Source: CAD feature listing. Evaluate the final solid. Frame: model axes, mm. A direction names the side the tool comes from. Round coordinates to 2 decimals unless told otherwise and drop trailing zeros. Write each loop counter-clockwise with the first axis right and the second up, starting at its lowest first coordinate (ties: lowest second). Pieces come first, ordered by that corner, then holes. Notation, with made-up numbers: (-10.75, -31.5) -> (3.25, -31.5) arc R20 ccw to (3.25, -6.5) -> close; hole circle Ø9 at (89, 87). An arc over 180 degrees is marked (long way). Return JSON: item names as keys, results as strings. Group by question number.
from build123d import *

# Parameters (mm, degrees)
F0_W     = 5.08
F0_H     = 5.08
F1_DEPTH = 5.08


# Not quite as in the source:
# - a feature names something its author has since deleted; it is built from what else it names


with BuildPart() as f1:
    # F0 (on Front) → F1 (new body)
    with BuildSketch(Plane.XZ):
        Polygon((0, 5.08), (0, 10.16), (-76.2, 10.16), (-76.2, 5.08), (-71.12, 5.08), (-71.12, 0), (-66.04, 0), (-66.04, -5.08), (-60.96, -5.08), (-60.96, -10.16), (-55.88, -10.16), (-55.88, -15.24), (-20.32, -15.24), (-20.32, -10.16), (-15.24, -10.16), (-15.24, -5.08), (-10.16, -5.08), (-10.16, 0), (-5.08, 0), (-5.08, 5.08), align=None)
        with Locations((-48.26, -7.62)):
            Rectangle(F0_W, F0_H, mode=Mode.SUBTRACT)
        with Locations((-38.1, -7.62)):
            Rectangle(F0_W, F0_H, mode=Mode.SUBTRACT)
        with Locations((-58.42, 2.54)):
            Rectangle(F0_W, F0_H, mode=Mode.SUBTRACT)
        with Locations((-48.26, 2.54)):
            Rectangle(F0_W, F0_H, mode=Mode.SUBTRACT)
        Polygon((76.2, 10.16), (0, 10.16), (0, 5.08), (5.08, 5.08), (5.08, 0), (10.16, 0), (10.16, -5.08), (15.24, -5.08), (15.24, -10.16), (20.32, -10.16), (55.88, -10.16), (60.96, -10.16), (60.96, -5.08), (66.04, -5.08), (66.04, 0), (71.12, 0), (71.12, 5.08), (76.2, 5.08), align=None)
        with Locations((17.78, 2.54)):
            Rectangle(F0_W, F0_H, mode=Mode.SUBTRACT)
        with Locations((27.94, 2.54)):
            Rectangle(F0_W, F0_H, mode=Mode.SUBTRACT)
    extrude(amount=-F1_DEPTH)


solid = f1.part
Item 1: Cut plane D-D on x = -38.5. Output: boundary loops of the cut face in (y, z).
Item 2: Material intervals for probe 1 along X at (y, z) = (2.55, -5.5); probe 2 along X at (y, z) = (4.45, -0.5); probe 3 along X at (y, z) = (1.05, -12.25), sorted ascending.
Item 3: Pull-direction query (X, two-part tool) for faces 6 (the flat face through (76.2, 3, 8)), 7 (the flat face through (-38, 3, -5.08)), 8 (the flat face through (74, 3, 5.08)); classes: +X half, -X half, draft (parallel to the pull), parting line (faces both ways), or undercut.
Item 4: Cut plane B-B on z = 2.25. Output: boundary loops of the cut face in (x, y), and give its area (3 significant figures).
Item 5: First-contact query: pin 1 Ø2 at (y, z) = (2, -3) entering from +X; pin 2 Ø1.5 at (x, y) = (-8.5, 2.5) entering from -Z; pin 3 Ø3 at (y, z) = (2.5, 1) entering from -X. Flat tips, straight axial feed; report the tip coordinate or a pass-through.
Item 6: Cut plane C-C on y = 3.2. Give the number of separate pieces and of enclosed holes in the cut face, and give its area (3 significant figures).
Item 7: Set-up query: faces 1 (the flat face through (13, 3, -5.08)), 2 (the flat face through (-60.96, 3, -8)), 3 (the flat face through (63, 3, -5.08)), 4 (the flat face through (-38, 3, -15.24)), 5 (the flat face through (-48, 3, 5.08)). Return all of +Z, -Z, +X, -X, +Y, -Y with unobstructed straight access to the full face (end or side cutting, diameter ignored); none if empty.
Item 8: Cut plane A-A on x = 17. Output: boundary loops of the cut face in (y, z), and give its area (3 significant figures).
Here are the results:
{
 "1": {"outline": "(0, -15.24) -> (5.08, -15.24) -> (5.08, -10.16) -> (0, -10.16) -> close; (0, -5.08) -> (5.08, -5.08) -> (5.08, 10.16) -> (0, 10.16) -> close"},
 "2": {"probe 1": "x = -60.96 to -50.8, -45.72 to -40.64, -35.56 to -15.24, 15.24 to 60.96", "probe 2": "x = -66.04 to -10.16, 10.16 to 66.04", "probe 3": "x = -55.88 to -20.32"},
 "3": {"face 6": "+X half", "face 7": "undercut", "face 8": "draft"},
 "4": {"outline": "(-71.12, 0) -> (-60.96, 0) -> (-60.96, 5.08) -> (-71.12, 5.08) -> close; (-55.88, 0) -> (-50.8, 0) -> (-50.8, 5.08) -> (-55.88, 5.08) -> close; (-45.72, 0) -> (-5.08, 0) -> (-5.08, 5.08) -> (-45.72, 5.08) -> close; (5.08, 0) -> (15.24, 0) -> (15.24, 5.08) -> (5.08, 5.08) -> close; (20.32, 0) -> (25.4, 0) -> (25.4, 5.08) -> (20.32, 5.08) -> close; (30.48, 0) -> (71.12, 0) -> (71.12, 5.08) -> (30.48, 5.08) -> close", "area": "568 mm^2"},
 "5": {"pin 1": "stops at x = 66.04", "pin 2": "stops at z = 0", "pin 3": "stops at x = -71.12"},
 "6": {"separate pieces": "1", "enclosed holes": "6", "area": "2,500 mm^2"},
 "7": {"face 1": "-Z, +Y, -Y", "face 2": "-Z, -X, +Y, -Y", "face 3": "-Z, +X, +Y, -Y", "face 4": "-Z, +X, -X, +Y, -Y", "face 5": "+Y, -Y"},
 "8": {"outline": "(0, -10.16) -> (5.08, -10.16) -> (5.08, 0) -> (0, 0) -> close; (0, 5.08) -> (5.08, 5.08) -> (5.08, 10.16) -> (0, 10.16) -> close", "area": "77.4 mm^2"}
}
